Design review of the part shown in the three views and the two pictorial views. Dimensions are in mm from the part's minimum x, y and z. Give positions to 0.01 mm unless a question says otherwise; leave off trailing zeros. Write each loop counter-clockwise with the first axis right and the second up, starting at its lowest first coordinate (ties: lowest second). Pieces come first, ordered by that corner, then holes.
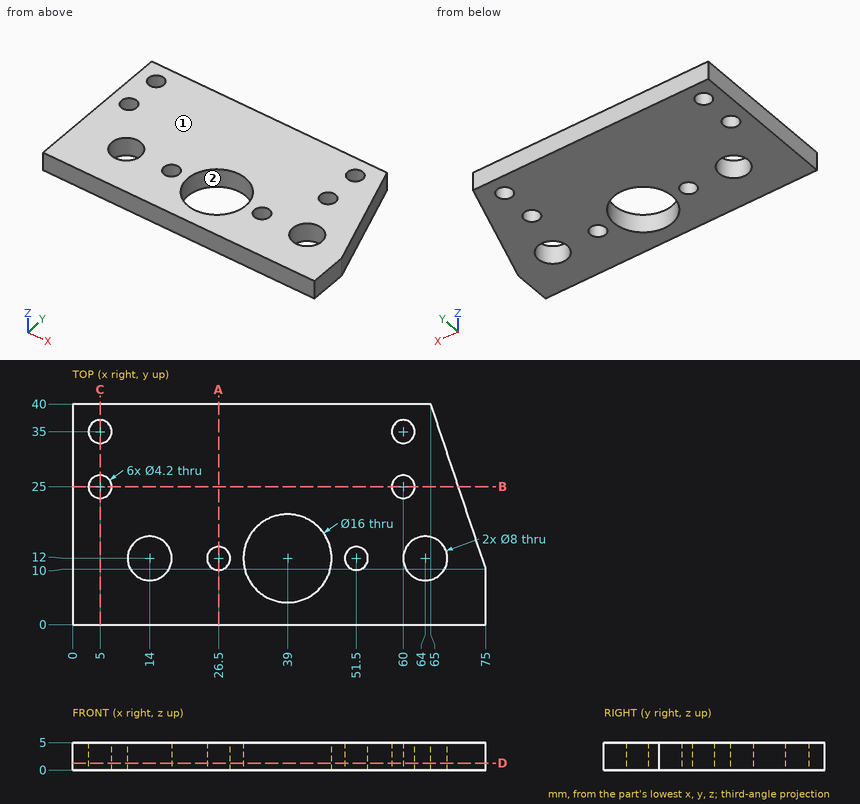
(1) Mouldability with a two-part tool opening along Y and no side actions: class the marked faces 1 and 2 as pulls with the +Y half, pulls with the -Y half, needs draft (parallel to the pull), parting line crosses it, or undercut.
Resolved:
face 1: needs draft
face 2: undercut
(2) Consider section A-A, the plane x = 26.5. Give the boundary of the cut face in (y, z), then the cut area to 3 significant figures.
Resolved:
outline: (0, 0) - (9.9, 0) - (9.9, 5) - (0, 5) - close; (14.1, 0) - (40, 0) - (40, 5) - (14.1, 5) - close
area: 179 mm2
(3) To check wall thickness, follow L1, parallel to Y at x = 5, z = 2.25; L2, parallel to X at y = 15.5, z = 3.1; L3, parallel to X at y = 10.5, z = 3.55. State the ranges of each line that lie inside material, in increasing order.
Resolved:
L1: y = 0 to 22.9, 27.1 to 32.9, 37.1 to 40
L2: x = 0 to 12.06, 15.94 to 31.81, 46.19 to 62.06, 65.94 to 73.17
L3: x = 0 to 10.29, 17.71 to 25.03, 27.97 to 31.14, 46.86 to 50.03, 52.97 to 60.29, 67.71 to 74.83
(4) Consider section D-D, the plane z = 1.25. Give the number of separate pieces and of enclosed holes in the cut face, then the cut area to 3 significant figures.
Resolved:
separate pieces: 1
enclosed holes: 9
area: 2,470 mm2
(5) Consider section B-B, the plane y = 25. Give the boundary of the cut face in (x, z), then the cut area to 3 significant figures.
Resolved:
outline: (0, 0) - (2.9, 0) - (2.9, 5) - (0, 5) - close; (7.1, 0) - (57.9, 0) - (57.9, 5) - (7.1, 5) - close; (62.1, 0) - (70, 0) - (70, 5) - (62.1, 5) - close
area: 308 mm2
(6) Consider section C-C, the plane x = 5. Give the boundary of the cut face in (y, z).
Resolved:
outline: (0, 0) - (22.9, 0) - (22.9, 5) - (0, 5) - close; (27.1, 0) - (32.9, 0) - (32.9, 5) - (27.1, 5) - close; (37.1, 0) - (40, 0) - (40, 5) - (37.1, 5) - close
